Could you check a few things on this model? Use its own coordinates, in mm. A direction names the side the tool comes from. Round coordinates to 2 decimals unless told otherwise and drop trailing zeros. Loops run counter-clockwise (first coordinate to the right, second up) from the corner with the lowest first, then second, coordinate; pieces in that order, holes last. Notation, with made-up numbers: (-24, -34) -> (8, -34) arc R20 ccw to (8, -5) -> close; hole circle Ø2 at (5, 30). An arc over 180 degrees is marked (long way). One line per item, written item: value.
```python
from build123d import *

# Parameters (mm, degrees)
SKETCH_R             = 80
SKETCH_R_2           = 15
SKETCH_R_3           = 1
PAD_DEPTH            = 3
SKETCH001_R          = 30
SKETCH001_R_2        = 27
PAD001_DEPTH         = 45
SKETCH002_R          = 6
PAD002_DEPTH         = 45
SKETCH004_R          = 1.6
POCKET_DEPTH         = 45.001
SKETCH003_R          = 4
POCKET001_DEPTH      = 20
SKETCH005_R          = 1
POCKET002_DEPTH      = 80.001
POCKET002_DEPTH_BACK = -80.001


with BuildPart() as part:
    # Sketch → Pad (new body)
    with BuildSketch(Plane.XY):
        Circle(SKETCH_R)
        Circle(SKETCH_R_2, mode=Mode.SUBTRACT)
        with Locations((-66.683956, 38.5)):
            Circle(SKETCH_R_3, mode=Mode.SUBTRACT)
        with Locations((66.683956, 38.5)):
            Circle(SKETCH_R_3, mode=Mode.SUBTRACT)
        with Locations((0, -77)):
            Circle(SKETCH_R_3, mode=Mode.SUBTRACT)
        with BuildLine():
            ThreePointArc((-15, 45), (0, 30), (15, 45))
            Line((15, 45), (15, 60))
            ThreePointArc((15, 60), (0, 75), (-15, 60))
            Line((-15, 45), (-15, 60))
        make_face(mode=Mode.SUBTRACT)
        with BuildLine():
            ThreePointArc((-31.471143, -35.490381), (-25.980762, -15), (-46.471143, -9.509619))
            Line((-46.471143, -9.509619), (-59.461524, -17.009619))
            ThreePointArc((-59.461524, -17.009619), (-64.951905, -37.5), (-44.461524, -42.990381))
            Line((-31.471143, -35.490381), (-44.461524, -42.990381))
        make_face(mode=Mode.SUBTRACT)
        with BuildLine():
            ThreePointArc((46.471143, -9.509619), (25.980762, -15), (31.471143, -35.490381))
            Line((31.471143, -35.490381), (44.461524, -42.990381))
            ThreePointArc((44.461524, -42.990381), (64.951905, -37.5), (59.461524, -17.009619))
            Line((46.471143, -9.509619), (59.461524, -17.009619))
        make_face(mode=Mode.SUBTRACT)
    extrude(amount=PAD_DEPTH)

    # Sketch001 → Pad001 (join)
    with BuildSketch(Plane.XY):
        Circle(SKETCH001_R)
        Circle(SKETCH001_R_2, mode=Mode.SUBTRACT)
    extrude(amount=PAD001_DEPTH)

    # Sketch002 → Pad002 (join)
    with BuildSketch(Plane.XY):
        with Locations((-20.78461, 12)):
            Circle(SKETCH002_R)
        with Locations((0, -24)):
            Circle(SKETCH002_R)
        with Locations((20.78461, 12)):
            Circle(SKETCH002_R)
    extrude(amount=PAD002_DEPTH)

    # Sketch004 → Pocket (cut, through all)
    with BuildSketch(Plane.XY):
        with Locations((-20.78461, 12)):
            Circle(SKETCH004_R)
        with Locations((20.78461, 12)):
            Circle(SKETCH004_R)
        with Locations((0, -24)):
            Circle(SKETCH004_R)
    extrude(amount=POCKET_DEPTH, mode=Mode.SUBTRACT)

    # Sketch003 → Pocket001 (cut)
    with BuildSketch(Plane.XY):
        with Locations((-20.78461, 12)):
            Circle(SKETCH003_R)
        with Locations((20.78461, 12)):
            Circle(SKETCH003_R)
        with Locations((0, -24)):
            Circle(SKETCH003_R)
    extrude(amount=POCKET001_DEPTH, mode=Mode.SUBTRACT)

    # Sketch005 → Pocket002 (cut, two sides)
    with BuildSketch(Plane.YZ) as pocket002_sk:
        with Locations((-28, 40)):
            Circle(SKETCH005_R)
    extrude(amount=-POCKET002_DEPTH, mode=Mode.SUBTRACT)
    extrude(pocket002_sk.sketch, amount=-POCKET002_DEPTH_BACK, mode=Mode.SUBTRACT)


solid = part.part
```
(1) Imagine slicing it at C-C on x = -49. Write out the boundary of the cut face in (y, z), then the cut area to 3 significant figures.
Results below:
outline: (-63.24, 0) -> (-44.7, 0) -> (-44.7, 3) -> (-63.24, 3) -> close; (-10.97, 0) -> (63.24, 0) -> (63.24, 3) -> (-10.97, 3) -> close
area: 278 mm²
(2) Imagine slicing it at D-D on z = 18. Write out the boundary of the cut face in (x, y).
Results below:
outline: circle Ø60 at (0, 0); hole (-25.64, 8.47) arc R27 ccw to (-5.48, -26.44) arc R6 cw (long way) to (5.48, -26.44) arc R27 ccw to (25.64, 8.47) arc R6 cw (long way) to (20.15, 17.97) arc R27 ccw to (-20.15, 17.97) arc R6 cw (long way) to start; hole circle Ø8 at (-20.78, 12); hole circle Ø8 at (0, -24); hole circle Ø8 at (20.78, 12)
(3) We'd pull the mould along X, two halves only. Please class faces 4 (the face through (-16, 9, 45)), 5 (the face through (-15.67, 8.86, 23.71)), 6 (the face through (-29.97, 1.32, 23.71)): +X half, -X half, draft (parallel to the pull), parting line (faces both ways), or undercut.
Results below:
face 4: draft
face 5: undercut
face 6: parting line
(4) On a 3-axis mill with a long thin cutter (end or side, diameter ignored), from which of +Z, -Z, +X, -X, +Y, -Y can I reach the whole of each face in a straight line? I mean faces 1 (the face through (34, 1, 3)), 2 (the face through (52.88, -13.21, 1.48)), 3 (the face through (-0.521, -20.034, 9.86)). Say none if no direction works.
Results below:
face 1: +Z
face 2: +Z, -Z
face 3: -Z
(5) For pin 1 Ø5 at (x, y) = (0, -24) entering from -Z; pin 2 Ø3 at (x, y) = (20.78, 12) entering from +Z; pin 3 Ø1 at (y, z) = (-24.5, 40.5) entering from -X; pin 4 Ø3.5 at (y, z) = (56, 1.5) entering from +X, each with a flat end and sliding along its axis, tell me the tip position at first contact or that it passes through.
Results below:
pin 1: stops at z = 20
pin 2: passes through
pin 3: stops at x = -18
pin 4: stops at x = 58.8
(6) Please list where these lines run through material, in increasing order: L1, parallel to Y at x = 0, z = 1.65; L2, parallel to Y at x = 0, z = 4.5; L3, parallel to Y at x = 2.5, z = 2.5.
Results below:
L1: y = -80 to -78, -76 to -28, -20 to -15, 15 to 30, 75 to 80
L2: y = -30 to -28, -20 to -18, 27 to 30
L3: y = -79.96 to -27.12, -20.88 to -14.79, 14.79 to 30.21, 74.79 to 79.96
(7) Imagine slicing it at B-B on y = 24. Write out the boundary of the cut face in (x, z).
Results below:
outline: (-76.32, 0) -> (76.32, 0) -> (76.32, 3) -> (18, 3) -> (18, 45) -> (12.37, 45) -> (12.37, 3) -> (-12.37, 3) -> (-12.37, 45) -> (-18, 45) -> (-18, 3) -> (-76.32, 3) -> close
(8) Imagine slicing it at A-A on z = 28. Write out the boundary of the cut face in (x, y).
Results below:
outline: circle Ø60 at (0, 0); hole (-25.64, 8.47) arc R27 ccw to (-5.48, -26.44) arc R6 cw (long way) to (5.48, -26.44) arc R27 ccw to (25.64, 8.47) arc R6 cw (long way) to (20.15, 17.97) arc R27 ccw to (-20.15, 17.97) arc R6 cw (long way) to start; hole circle Ø3.2 at (-20.78, 12); hole circle Ø3.2 at (0, -24); hole circle Ø3.2 at (20.78, 12)
